from build123d import *

# Parameters (mm, degrees)
AUFSATZ_LINEAR_AUSTRAGEN1_DEPTH      = 18
F_16_0_16_DURCHMESSER_BOHRUNG1_D     = 16
F_16_0_16_DURCHMESSER_BOHRUNG1_DEPTH = 13
F_16_0_16_DURCHMESSER_BOHRUNG1_TIP   = 4.806884952
F_1_75_1_75_DURCHMESSER_BOHRUNG1_D   = 1.75


with BuildPart() as part:
    # Skizze1 → Aufsatz-Linear austragen1 (new body)
    with BuildSketch(Plane.XY):
        Polygon((15.011106999, 0), (7.505553499, 13), (-7.505553499, 13), (-15.011106999, 0), (-7.505553499, -13), (7.505553499, -13), align=None)
    extrude(amount=AUFSATZ_LINEAR_AUSTRAGEN1_DEPTH)

    # Ø16.0 (16) Durchmesser Bohrung1
    with Locations(Plane(origin=(0, 0, 0), x_dir=(-1, 0, 0), z_dir=(0, 0, -1))):
        with Locations((0, 0)):
            Hole(F_16_0_16_DURCHMESSER_BOHRUNG1_D / 2, depth=F_16_0_16_DURCHMESSER_BOHRUNG1_DEPTH)
            with Locations((0, 0, -(F_16_0_16_DURCHMESSER_BOHRUNG1_DEPTH + F_16_0_16_DURCHMESSER_BOHRUNG1_TIP / 2))):  # 118° drill point
                Cone(0, F_16_0_16_DURCHMESSER_BOHRUNG1_D / 2, F_16_0_16_DURCHMESSER_BOHRUNG1_TIP, mode=Mode.SUBTRACT)

    # Ø1.75 (1.75) Durchmesser Bohrung1 (through all)
    with Locations(Plane.XY.offset(18)):
        with Locations((0, 0)):
            Hole(F_1_75_1_75_DURCHMESSER_BOHRUNG1_D / 2)


solid = part.part
The listing builds one solid part. Answer for the finished solid, in the listing's coordinates (mm). A direction names the side the tool comes from. Give positions to 0.01 mm unless a question says otherwise; leave off trailing zeros. Write each loop counter-clockwise with the first axis right and the second up, starting at its lowest first coordinate (ties: lowest second). Pieces come first, ordered by that corner, then holes. Notation, with made-up numbers: (42.5, -35) -> (90.5, -35) arc R18 cw to (90.5, -11) -> close; hole circle Ø8 at (61, 84.25). An arc over 180 degrees is marked (long way). Use a Markdown table: item, result.
(1) Flat-ended cylindrical pins translate along their axes: P1, Ø8, axis at y = -3.5, z = 7, coming from the -X side; P2, Ø2, axis at y = -10, z = 10.5, coming from the -X side; P3, Ø8, axis at y = 7.5, z = 11.5, coming from the +X side. Find the tip coordinate at first contact, or state that the pin passes through.
Return value:
| item | result |
|---|---|
| P1 | x = -15.01 |
| P2 | x = -9.81 |
| P3 | x = 12.99 |
(2) Section B-B, the plane z = 4.75 is taken. Determine the outline of the cut face in (x, y), then the cut area to 3 significant figures.
Return value:
| item | result |
|---|---|
| outline | (-15.01, 0) -> (-7.51, -13) -> (7.51, -13) -> (15.01, 0) -> (7.51, 13) -> (-7.51, 13) -> close; hole circle Ø16 at (0, 0) |
| area | 384 mm2 |
(3) Find the intervals of material crossed by probe 1 along Y at (x, z) = (0, 3.5); probe 2 along X at (y, z) = (0, 6.5); probe 3 along X at (y, z) = (-5, 4) (3 decimals), in increasing order. Write a range as from..to.
Return value:
| item | result |
|---|---|
| probe 1 | -13..-8, 8..13 |
| probe 2 | -15.01..-8, 8..15.01 |
| probe 3 | -12.124..-6.245, 6.245..12.124 |
(4) Determine the mould class of faces 1 (the flat face through (6, 6, 0)), 2 (the flat face through (11.2, -6.6, 8.9)), 3 (the conical face through (-1.26, 0.397, 17.013)) for opening direction X: released by +X, released by -X, zero draft, split by the parting line, or undercut.
Return value:
| item | result |
|---|---|
| face 1 | zero draft |
| face 2 | released by +X |
| face 3 | undercut |
(5) Section C-C, the plane z = 13.5 is taken. Determine the outline of the cut face in (x, y).
Return value:
| item | result |
|---|---|
| outline | (-15.01, 0) -> (-7.51, -13) -> (7.51, -13) -> (15.01, 0) -> (7.51, 13) -> (-7.51, 13) -> close; hole circle Ø14.34 at (0, 0) |
(6) Section D-D, the plane y = 11 is taken. Determine the outline of the cut face in (x, z), then the cut area to 3 significant figures.
Return value:
| item | result |
|---|---|
| outline | (-8.66, 0) -> (8.66, 0) -> (8.66, 18) -> (-8.66, 18) -> close |
| area | 312 mm2 |
(7) Section A-A, the plane x = 0 is taken. Determine the outline of the cut face in (y, z) (3 decimals).
Return value:
| item | result |
|---|---|
| outline | (-13, 0) -> (-8, 0) -> (-8, 13) -> (-0.875, 17.281) -> (-0.875, 18) -> (-13, 18) -> close; (0.875, 17.281) -> (8, 13) -> (8, 0) -> (13, 0) -> (13, 18) -> (0.875, 18) -> close |
(8) For faces 4 (the flat face through (0, -13, 9)), 5 (the cylindrical face through (-1.73, -7.81, 6.59)), determine the directions among +Z, -Z, +X, -X, +Y, -Y from which every point of the face is accessible in a straight line to the end or side of a thin tool.
Return value:
| item | result |
|---|---|
| face 4 | +Z, -Z, +X, -X, -Y |
| face 5 | -Z |
